Design review of the part built by this model. Coordinates are the model's own, in mm. A direction names the side the tool comes from. Coordinates: 2 decimals unless noted, no trailing zeros. Write each loop counter-clockwise with the first axis right and the second up, starting at its lowest first coordinate (ties: lowest second). Pieces come first, ordered by that corner, then holes. Notation, with made-up numbers: (82.5, -6) - (102.5, -6) arc R22 cw to (102.5, 32) - close; hole circle Ø2 at (50.25, 62). An arc over 180 degrees is marked (long way). One line per item, written item: value.
from build123d import *
from build123d.topology import SkipClean

# Parameters (mm, degrees)
SKETCH1_W               = 19.20875
SKETCH1_H               = 68.2625
SKETCH2_W               = 19.20875
SKETCH2_H               = 37.94125
SKETCH7_R               = 15.875
CUT_EXTRUDE1_DEPTH      = 81.425639161
CUT_EXTRUDE2_REACH      = 71.282
CUT_EXTRUDE2_END_RADIUS = 15.875
SKETCH8_R               = 15.875
SKETCH9_R               = 16.66875
CUT_EXTRUDE3_DEPTH      = 19.05
CUT_EXTRUDE4_START      = -19.05
SKETCH10_R              = 16.66875
CUT_EXTRUDE4_DEPTH      = 19.05
SKETCH11_R              = 16.66875
CUT_EXTRUDE5_DEPTH      = 19.05


with BuildPart() as part:
    # Sketch1 → Revolve1 (revolve)
    with BuildSketch(Plane(origin=(0, 0, 0), x_dir=(1, 0, 0), z_dir=(0, 1, 0)), mode=Mode.PRIVATE) as revolve1_sk:
        with Locations((9.604375, 0)):
            Rectangle(SKETCH1_W, SKETCH1_H)
    revolve(revolve1_sk.sketch.rotate(Axis((0, 0, 118.243982537), (0, 0, -1)), 180), axis=Axis((0, 0, 118.243982537), (0, 0, -1)))

    # Sketch2 → Revolve2 (revolve)
    with BuildSketch(Plane.XY, mode=Mode.PRIVATE) as revolve2_sk:
        with Locations((-9.604375, 18.970625)):
            Rectangle(SKETCH2_W, SKETCH2_H)
    revolve(revolve2_sk.sketch.rotate(Axis((0, 0, 0), (0, 1, 0)), 90), axis=Axis((0, 0, 0), (0, 1, 0)))

    # Sketch7 → Cut-Extrude1 (cut, through all)
    with BuildSketch(Plane.XY.offset(34.13125)):
        Circle(SKETCH7_R)
    extrude(amount=-CUT_EXTRUDE1_DEPTH, mode=Mode.SUBTRACT)

    # Cut-Extrude2: up to this cylinder (the profile starts outside it)
    cut_extrude2_end = Plane(origin=(0, 0, 0), z_dir=(0, 0, 1)) * Cylinder(CUT_EXTRUDE2_END_RADIUS, 175.314, mode=Mode.PRIVATE)
    # Sketch8 → Cut-Extrude2 (cut, up to the surface)
    with BuildSketch(Plane(origin=(0, 37.94125, 0), x_dir=(1, 0, 0), z_dir=(0, 1, 0)), mode=Mode.PRIVATE) as cut_extrude2_sk1:
        with Locations(Location((0, 0, 0), (0, 0, 270))):
            Circle(SKETCH8_R)
    cut_extrude2_tool1 = extrude(cut_extrude2_sk1.sketch, amount=-CUT_EXTRUDE2_REACH, mode=Mode.PRIVATE) - cut_extrude2_end
    add(cut_extrude2_tool1.solids().sort_by_distance((0, 37.94125, 0))[0], mode=Mode.SUBTRACT)

    # Sketch9 → Cut-Extrude3 (cut)
    with SkipClean():  # the faces are left unmerged after this step: merging them gives an invalid solid
        with BuildSketch(Plane.XY.offset(34.13125)):
            Circle(SKETCH9_R)
        extrude(amount=-CUT_EXTRUDE3_DEPTH, mode=Mode.SUBTRACT)

    # Sketch10 → Cut-Extrude4 (cut)
    with BuildSketch(Plane(origin=(0, 0, -34.13125), x_dir=(-1, 0, 0), z_dir=(0, 0, -1)).offset(CUT_EXTRUDE4_START)):
        with Locations(Location((0, 0, 0), (0, 0, 180))):
            Circle(SKETCH10_R)
    extrude(amount=CUT_EXTRUDE4_DEPTH, mode=Mode.SUBTRACT)

    # Sketch11 → Cut-Extrude5 (cut)
    with BuildSketch(Plane(origin=(0, 37.94125, 0), x_dir=(1, 0, 0), z_dir=(0, 1, 0))):
        with Locations(Location((0, 0, 0), (0, 0, 270))):
            Circle(SKETCH11_R)
    extrude(amount=-CUT_EXTRUDE5_DEPTH, mode=Mode.SUBTRACT)


solid = part.part
1. Wall thickness on line 1 along X through (y, z) = (0, 20); line 2 along X through (y, z) = (10, 0) (3 decimals): over which ranges is each line inside the solid? List them lowest first.
Answer block:
line 1: x = -19.21 to -16.67, 16.67 to 19.21
line 2: x = -19.209 to -15.875, 15.875 to 19.209
2. Insertion check: pin 1 Ø10 at (x, y) = (-1, 25) entering from +Z; pin 2 Ø1.5 at (x, z) = (10, 0) entering from -Y; pin 3 Ø3 at (y, z) = (21, 11.5) entering from -X. Each pin has a flat end and moves straight along its axis. Give the tip position at first contact, or say it passes through.
Answer block:
pin 1: stops at z = 19.21
pin 2: stops at y = -16.83
pin 3: stops at x = -16.4
3. Consider section A-A, the plane x = 0. Write out the cut boundary in (y, z) (3 decimals).
Answer block:
outline: (-19.209, -34.131) - (-16.669, -34.131) - (-16.669, -15.081) - (-15.875, -15.081) - (-15.875, 15.081) - (-16.669, 15.081) - (-16.669, 34.131) - (-19.209, 34.131) - close; (16.669, -34.131) - (19.209, -34.131) - (19.209, -19.209) - (37.941, -19.209) - (37.941, -16.669) - (18.891, -16.669) - (18.891, -15.875) - (16.669, -15.875) - close; (16.669, 15.875) - (18.891, 15.875) - (18.891, 16.669) - (37.941, 16.669) - (37.941, 19.209) - (19.209, 19.209) - (19.209, 34.131) - (16.669, 34.131) - close
4. Consider section D-D, the plane x = 13.5. Write out the cut boundary in (y, z).
Answer block:
outline: (-13.66, -34.13) - (-9.78, -34.13) - (-9.78, -15.08) - (-8.35, -15.08) - (-8.35, 15.08) - (-9.78, 15.08) - (-9.78, 34.13) - (-13.66, 34.13) - close; (8.35, -15.08) - (9.78, -15.08) - (9.78, -34.13) - (13.66, -34.13) - (13.66, -13.66) - (37.94, -13.66) - (37.94, -9.78) - (18.89, -9.78) - (18.89, -8.35) - (8.35, -8.35) - close; (8.35, 8.35) - (18.89, 8.35) - (18.89, 9.78) - (37.94, 9.78) - (37.94, 13.66) - (13.66, 13.66) - (13.66, 34.13) - (9.78, 34.13) - (9.78, 15.08) - (8.35, 15.08) - close
5. Mouldability with a two-part tool opening along X and no side actions: class faces 1 (the face through (-6, 16, 34.131)), 2 (the face through (-1, -16, 15.081)), 3 (the face through (16.197, 23.452, 10.327)) as released by +X, released by -X, zero draft, split by the parting line, or undercut.
Answer block:
face 1: zero draft
face 2: undercut
face 3: split by the parting line
6. For faces 4 (the face through (15.9, -5, -24.5)), 5 (the face through (5, 28.5, 15.9)), 6 (the face through (4.164, -18.752, -0.478)), 7 (the face through (15.9, 5, 24.7)), list the 3-axis set-ups (+Z, -Z, +X, -X, +Y, -Y) from which the entire face can be reached by the end or side of a thin tool; tool diameter is ignored.
Answer block:
face 4: -Z
face 5: +Y
face 6: none
face 7: +Z
